Geometry check sheet. Reference: the model listing, model coordinates, mm. Round coordinates to 2 decimals unless told otherwise and drop trailing zeros. Order: outer loops, then holes, each group sorted by start corner. A loop starts at its lowest first (then second) coordinate and runs counter-clockwise, first axis right, second up. Notation, with made-up numbers: (71.5, -31.75) -> (126.5, -31.75) arc R33 ccw to (126.5, 1.25) -> close; hole circle Ø2 at (46, 57). An arc over 180 degrees is marked (long way). Answer as a JSON object with one key per item and string values. Group by question number.
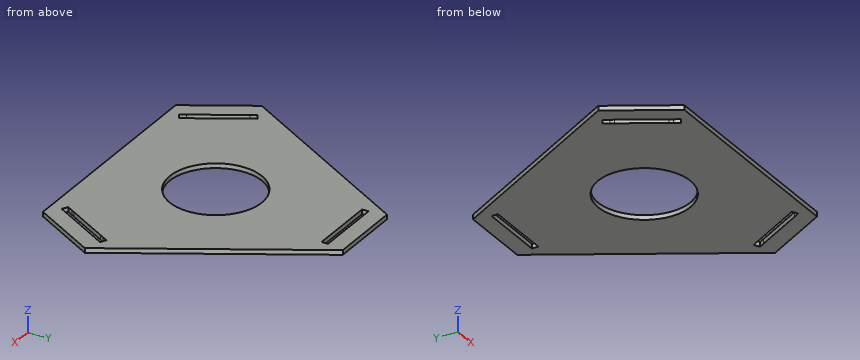
from build123d import *

# Parameters (mm, degrees)
SKETCH1_R           = 50
BOSS_EXTRUDE1_DEPTH = 5


with BuildPart() as part:
    # Sketch1 → Boss-Extrude1 (new body)
    with BuildSketch(Plane.XY):
        Polygon((0, 0), (240, 0), (280, 69.282032303), (160, 277.128129211), (80, 277.128129211), (-40, 69.282032303), align=None)
        with Locations((120, 115.470053838)):
            Circle(SKETCH1_R, mode=Mode.SUBTRACT)
        Polygon((149.607695155, 259.128129211), (90.392304845, 259.128129211), (83.392304845, 259.128129211), (83.392304845, 252.128129211), (90.392304845, 252.128129211), (94.43375673, 252.128129211), (145.56624327, 252.128129211), (149.607695155, 252.128129211), (156.607695155, 252.128129211), (156.607695155, 259.128129211), align=None, mode=Mode.SUBTRACT)
        Polygon((225.56624327, 25), (251.132486541, 69.282032303), (253.153212483, 72.782032303), (256.653212483, 78.844210129), (262.715390309, 75.344210129), (259.215390309, 69.282032303), (229.607695155, 18), (226.107695155, 11.937822174), (220.045517328, 15.437822174), (223.545517328, 21.5), align=None, mode=Mode.SUBTRACT)
        Polygon((-11.132486541, 69.282032303), (14.43375673, 25), (16.454482672, 21.5), (19.954482672, 15.437822174), (13.892304845, 11.937822174), (10.392304845, 18), (-19.215390309, 69.282032303), (-22.715390309, 75.344210129), (-16.653212483, 78.844210129), (-13.153212483, 72.782032303), align=None, mode=Mode.SUBTRACT)
    extrude(amount=BOSS_EXTRUDE1_DEPTH)


solid = part.part
Item 1: Sectioned sample at C-C, the plane z = 2.3. Enter the section's corners in (x, y), then the cut area to 3 significant figures.
Item 2: Sectioned sample at A-A, the plane x = 120. Enter the section's corners in (y, z), then the cut area to 3 significant figures.
Item 3: Depth check by flat-ended pin: pin 1 Ø1.5 at (y, z) = (256, 3.5) entering from +X; pin 2 Ø3 at (y, z) = (55, 2) entering from -X; pin 3 Ø8 at (x, y) = (189.5, 90) entering from -Z; pin 4 Ø10 at (x, y) = (94.5, 79) entering from -Z. Enter the tip coordinate at first touch or a pass-through.
Item 4: Thickness scan on L1, parallel to Y at x = 120, z = 3.25; L2, parallel to Y at x = 121.5, z = 2.2; L3, parallel to X at y = 25, z = 2.9. Record the ranges inside material, lowest first.
Item 5: Sectioned sample at B-B, the plane y = 33.5. Enter the section's corners in (x, z), then the cut area to 3 significant figures.
Item 6: Sectioned sample at D-D, the plane y = 120. Enter the section's corners in (x, z), then the cut area to 3 significant figures.
Result:
{
 "1": {"outline": "(-40, 69.28) -> (0, 0) -> (240, 0) -> (280, 69.28) -> (160, 277.13) -> (80, 277.13) -> close; hole (-22.72, 75.34) -> (13.89, 11.94) -> (19.95, 15.44) -> (-16.65, 78.84) -> close; hole circle Ø100 at (120, 115.47); hole (83.39, 252.13) -> (156.61, 252.13) -> (156.61, 259.13) -> (83.39, 259.13) -> close; hole (220.05, 15.44) -> (226.11, 11.94) -> (262.72, 75.34) -> (256.65, 78.84) -> close", "area": "51,600 mm2"},
 "2": {"outline": "(0, 0) -> (65.47, 0) -> (65.47, 5) -> (0, 5) -> close; (165.47, 0) -> (252.13, 0) -> (252.13, 5) -> (165.47, 5) -> close; (259.13, 0) -> (277.13, 0) -> (277.13, 5) -> (259.13, 5) -> close", "area": "851 mm2"},
 "3": {"pin 1": "stops at x = 172.63", "pin 2": "stops at x = -32.62", "pin 3": "stops at z = 0", "pin 4": "passes through"},
 "4": {"L1": "y = 0 to 65.47, 165.47 to 252.13, 259.13 to 277.13", "L2": "y = 0 to 65.49, 165.45 to 252.13, 259.13 to 277.13", "L3": "x = -14.43 to 6.35, 14.43 to 225.57, 233.65 to 254.43"},
 "5": {"outline": "(-19.34, 0) -> (1.44, 0) -> (1.44, 5) -> (-19.34, 5) -> close; (9.53, 0) -> (230.47, 0) -> (230.47, 5) -> (9.53, 5) -> close; (238.56, 0) -> (259.34, 0) -> (259.34, 5) -> (238.56, 5) -> close", "area": "1,310 mm2"},
 "6": {"outline": "(-10.72, 0) -> (70.21, 0) -> (70.21, 5) -> (-10.72, 5) -> close; (169.79, 0) -> (250.72, 0) -> (250.72, 5) -> (169.79, 5) -> close", "area": "809 mm2"}
}
